Could you check a few things on this model? Use its own coordinates, in mm. A direction names the side the tool comes from. Coordinates: 2 decimals unless noted, no trailing zeros. Write each loop counter-clockwise with the first axis right and the second up, starting at its lowest first coordinate (ties: lowest second). Pieces come first, ordered by that corner, then holes. Notation, with made-up numbers: (-17, 32) - (36, 32) arc R15 ccw to (36, 57) - close; hole circle Ø1 at (-32.75, -7.75). An arc over 180 degrees is marked (long way). Answer as a JSON object with one key per item and string values. Group by question number.
1) On a 3-axis mill with a long thin cutter (end or side, diameter ignored), from which of +Z, -Z, +X, -X, +Y, -Y can I reach the whole of each face in a straight line? I mean faces 5 (the cylindrical face through (6.596, 3.131, 8.875)), 6 (the flat face through (19.05, 3, 17)). Say none if no direction works.
2) If we section it at A-A (y = 5): Write out the boundary of the cut face in (x, z) (3 decimals).
3) Will these pins go through, and if not, where does the flat tip stop? pin 1 Ø3 at (y, z) = (3, 17.5) entering from +X; pin 2 Ø3 at (y, z) = (4, 14.5) entering from -X; pin 3 Ø1 at (y, z) = (5, 77.5) entering from -X.
4) We'd pull the mould along X, two halves only. Please class faces 1 (the flat face through (-18, 0, 56)), 2 (the cylindrical face through (-11.78, 3.13, 103.19)), 3 (the flat face through (0, 3, 13)), 4 (the cylindrical face through (16.733, 3.131, 29.13)): released by +X, released by -X, zero draft, split by the parting line, or undercut.
5) If we section it at D-D (x = -21.5): Write out the boundary of the cut face in (y, z), plus the area to 3 significant figures.
6) If we section it at C-C (z = 91): Write out the boundary of the cut face in (x, y).
7) If we section it at B-B (x = -2.5): Write out the boundary of the cut face in (y, z).
8) Please list where these lines run through material, in increasing order: line 1 along Z through (x, y) = (-14, 6) (3 decimals); line 2 along X through (y, z) = (2, 11); line 3 along Z through (x, y) = (16, 4.25).
```python
from build123d import *

# Parameters (mm, degrees)
SKETCH1_R           = 3
SKETCH1_R_2         = 2
BOSS_EXTRUDE1_DEPTH = 6.35
FILLET1_R           = 10.16


with BuildPart() as part:
    # Sketch1 → Boss-Extrude1 (new body)
    with BuildSketch(Plane(origin=(0, 0, 0), x_dir=(1, 0, 0), z_dir=(0, 1, 0))):
        with BuildLine():
            Line((19.05, 0), (0, 0))
            Line((0, 0), (0, -22.757139607))
            ThreePointArc((0, -22.757139607), (-30.814603217, -79.553676933), (19.05, -120.65))
            ThreePointArc((19.05, -120.65), (25.4, -114.3), (19.05, -107.95))
            ThreePointArc((19.05, -107.95), (-19.05, -69.85), (19.05, -31.75))
            Line((19.05, -31.75), (19.05, 0))
        make_face()
        with Locations(Location((9.525, -9.525, 0), (0, 0, 270))):
            Circle(SKETCH1_R, mode=Mode.SUBTRACT)
        with Locations(Location((-12.380896424, -38.419103576, 0), (0, 0, 270))):
            Circle(SKETCH1_R_2, mode=Mode.SUBTRACT)
        with Locations(Location((-12.380896424, -101.280896424, 0), (0, 0, 270))):
            Circle(SKETCH1_R_2, mode=Mode.SUBTRACT)
    extrude(amount=BOSS_EXTRUDE1_DEPTH)

    # Fillet1
    # the kernel refuses this fillet: 10.16 mm, written as the material it adds along each edge
    with BuildSketch(Plane(origin=(0, 0, 22.757139607), x_dir=(0, 0, -1), z_dir=(0, 1, 0))) as fillet1_piece_1:
        with BuildLine():
            CenterArc((6.413190667, 10.16), FILLET1_R, 208.630989837, 61.369010163)
            ThreePointArc((-2.50448451, 5.291666667), (-1.175949507, 2.681941807), (0, 0))
            Line((0, 0), (6.413190667, 0))
        make_face()
    extrude(amount=6.35)
    # the kernel refuses this fillet: 10.16 mm, written as the material it takes off along each edge
    with BuildSketch(Plane(origin=(19.05, -22.696015193, 31.75), x_dir=(0, 0, -1), z_dir=(0, 1, 0))) as fillet1_2_piece_1:
        with BuildLine():
            CenterArc((9.078406077, 10.16), FILLET1_R, 192.153197469, 77.846802531)
            ThreePointArc((-0.853889939, 8.021052632), (-0.214073897, 4.033187739), (0, 0))
            Line((0, 0), (9.078406077, 0))
        make_face()
    extrude(amount=51.742030387, mode=Mode.SUBTRACT)
    with BuildSketch(Plane(origin=(0, -25.4, 0), x_dir=(1, 0, 0), z_dir=(0, 1, 0)), Plane(origin=(19.05, -25.4, 0), x_dir=(0, 0, 1), z_dir=(0, 1, 0))) as fillet1_2_piece_2:
        with BuildLine():
            CenterArc((FILLET1_R, -FILLET1_R), FILLET1_R, 90, 90)
            Line((0, -FILLET1_R), (0, 0))
            Line((0, 0), (FILLET1_R, 0))
        make_face()
    extrude(amount=57.15, mode=Mode.SUBTRACT)


solid = part.part
```
Here are the results:
{
 "1": {"face 5": "+Y, -Y", "face 6": "-Z, +X, +Y, -Y"},
 "2": {"outline": "(-5.292, 25.262) arc R10.16 cw to (0, 16.344) - (0, 10.16) arc R10.16 ccw to (9.525, 0.02) arc R10.16 ccw to (19.05, 10.16) - (19.05, 22.672) arc R10.16 ccw to (11.029, 32.604) arc R38.1 cw to (19.05, 107.95) arc R6.35 ccw to (19.05, 120.65) arc R50.8 ccw to start; hole circle Ø4 at (-12.381, 38.419); hole circle Ø4 at (-12.381, 101.281); hole circle Ø6 at (9.525, 9.525)"},
 "3": {"pin 1": "stops at x = 19.05", "pin 2": "stops at x = 0", "pin 3": "stops at x = -31.24"},
 "4": {"face 1": "zero draft", "face 2": "undercut", "face 3": "released by -X", "face 4": "released by +X"},
 "5": {"outline": "(0, 39.25) - (6.35, 39.25) - (6.35, 100.45) - (0, 100.45) - close", "area": "389 mm²"},
 "6": {"outline": "(-27.14, 0) - (-12.64, 0) - (-12.64, 6.35) - (-27.14, 6.35) - close"},
 "7": {"outline": "(0, 23.02) - (6.35, 23.02) - (6.35, 38.43) - (0, 38.43) - close; (0, 101.27) - (6.35, 101.27) - (6.35, 115.85) - (0, 115.85) - close"},
 "8": {"line 1": "z = 31.271 to 37.245, 39.593 to 50.895, 88.805 to 100.107, 102.455 to 108.429", "line 2": "x = 0 to 6.91, 12.14 to 19.05", "line 3": "z = 2.9 to 29.93, 107.83 to 120.56"}
}
